Geometry: final body of the model. Coordinates: model frame, mm. Give positions to 0.01 mm unless a question says otherwise; leave off trailing zeros. Loops run counter-clockwise (first coordinate to the right, second up) from the corner with the lowest first, then second, coordinate; pieces in that order, holes last. Notation, with made-up numbers: (32.25, 34.25) -> (64.25, 34.25) arc R22 cw to (64.25, 45.25) -> close; hole circle Ø6 at (-30, 0). An arc over 180 degrees is marked (long way). Answer in a Markdown table with one row per item. Add a question column.
1) First-contact query: P1, Ø3.5, axis at y = 8.5, z = 14.5, coming from the +X side; P2, Ø3.5, axis at x = -110.5, y = 6, coming from the -Z side; P3, Ø6, axis at x = -112.5, y = 5.5, coming from the +Z side. Flat tips, straight axial feed; report the tip coordinate or a pass-through.
2) Section query B-B (x = 3). Return the cut outline in (y, z), plus the area to 3 significant figures.
3) Line query: line 1 (X direction, y = 4, z = -3.5); line 2 (Z direction, x = -16.5, y = 9); line 3 (X direction, y = 5.75, z = -119). Output: solid intervals per line, ascending. Write a range as from..to.
4) Section query A-A (z = -85). Return the cut outline in (x, y), plus the area to 3 significant figures.
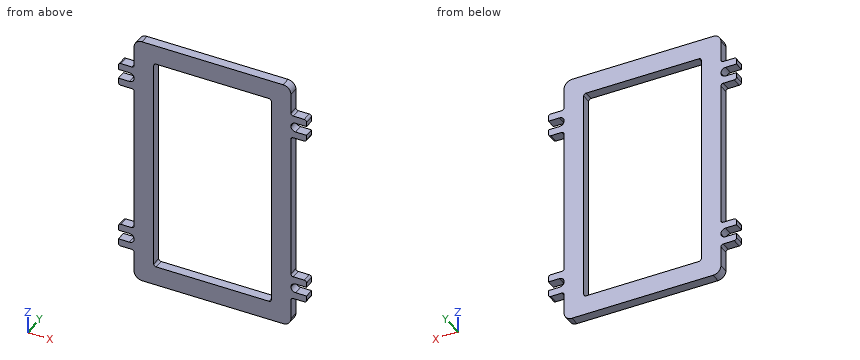
```python
from build123d import *

# Parameters (mm, degrees)
BOSS_EXTRUDE1_DEPTH  = 12
BOSS_EXTRUDE2_DEPTH  = 12
MIRROR4_COPY_1_DEPTH = 12
FILLET3_R            = 6
FILLET4_R            = 3


with BuildPart() as part:
    # Sketch2 → Boss-Extrude1 (new body)
    with BuildSketch(Plane(origin=(0, 0, 0), x_dir=(1, 0, 0), z_dir=(0, 1, 0))):
        with BuildLine():
            Line((-90, -165), (90, -165))
            ThreePointArc((90, -165), (97.071067812, -162.071067812), (100, -155))
            Line((100, -155), (100, 155))
            ThreePointArc((100, 155), (97.071067812, 162.071067812), (90, 165))
            Line((90, 165), (-90, 165))
            ThreePointArc((-90, 165), (-97.071067812, 162.071067812), (-100, 155))
            Line((-100, 155), (-100, -155))
            ThreePointArc((-100, -155), (-97.071067812, -162.071067812), (-90, -165))
        make_face()
        with BuildLine():
            Line((-72, -140), (72, -140))
            ThreePointArc((72, -140), (74.121320344, -139.121320344), (75, -137))
            Line((75, -137), (75, 137))
            ThreePointArc((75, 137), (74.121320344, 139.121320344), (72, 140))
            Line((72, 140), (-72, 140))
            ThreePointArc((-72, 140), (-74.121320344, 139.121320344), (-75, 137))
            Line((-75, 137), (-75, -137))
            ThreePointArc((-75, -137), (-74.121320344, -139.121320344), (-72, -140))
        make_face(mode=Mode.SUBTRACT)
    extrude(amount=BOSS_EXTRUDE1_DEPTH)

    # Sketch3 → Boss-Extrude2 (add)
    with BuildSketch(Plane(origin=(0, 0, 0), x_dir=(1, 0, 0), z_dir=(0, 1, 0))):
        Polygon((75, 126), (120, 126), (120, 117), (97, 117), (97, 105), (120, 105), (120, 96), (75, 96), align=None)
    boss_extrude2 = extrude(amount=BOSS_EXTRUDE2_DEPTH)

    # Mirror3: Boss-Extrude2 across plane
    add(boss_extrude2.mirror(Plane(origin=(0, 0, 0), x_dir=(0, 0, 1), z_dir=(1, 0, 0))))

    # Mirror4: Boss-Extrude2 across plane
    add(boss_extrude2.mirror(Plane.XY))

    # Mirror4 copy 1 sketch → Mirror4 copy 1 (add)
    with BuildSketch(Plane(origin=(0, 0, 0), x_dir=(-1, 0, 0), z_dir=(0, 1, 0))):
        Polygon((75, 126), (120, 126), (120, 117), (97, 117), (97, 105), (120, 105), (120, 96), (75, 96), align=None)
    extrude(amount=MIRROR4_COPY_1_DEPTH)

    # Fillet3
    fillet3_edges = [part.edges().sort_by_distance(p)[0] for p in [
        (-100, 6, 117),
        (-100, 6, 105),
        (100, 6, 117),
        (100, 6, 105),
        (100, 6, -105),
        (100, 6, -117),
        (-100, 6, -105),
        (-100, 6, -117),
    ]]
    fillet(fillet3_edges, radius=FILLET3_R - 0.0001)  # a hair under: the kernel refuses the full size

    # Fillet4
    fillet4_edges = [part.edges().sort_by_distance(p)[0] for p in [
        (-120, 6, -96),
        (-120, 6, -126),
        (-100, 6, -96),
        (-100, 6, -126),
        (120, 6, 96),
        (120, 6, 126),
        (100, 6, 96),
        (100, 6, 126),
        (-100, 6, 126),
        (-120, 6, 126),
        (-100, 6, 96),
        (-120, 6, 96),
        (100, 6, -126),
        (120, 6, -126),
        (100, 6, -96),
        (120, 6, -96),
    ]]
    fillet(fillet4_edges, radius=FILLET4_R)


solid = part.part
```
Evaluation:
| question | item | result |
|---|---|---|
| 1 | P1 | x = 100 |
| 1 | P2 | z = -126 |
| 1 | P3 | z = 126 |
| 2 | outline | (0, -165) -> (12, -165) -> (12, -140) -> (0, -140) -> close; (0, 140) -> (12, 140) -> (12, 165) -> (0, 165) -> close |
| 2 | area | 600 mm² |
| 3 | line 1 | -100..-75, 75..100 |
| 3 | line 2 | -165..-140, 140..165 |
| 3 | line 3 | -120..-75, 75..120 |
| 4 | outline | (-100, 0) -> (-75, 0) -> (-75, 12) -> (-100, 12) -> close; (75, 0) -> (100, 0) -> (100, 12) -> (75, 12) -> close |
| 4 | area | 600 mm² |
